Work out the finished part from the listing and answer in its coordinate system (mm). Face numbers are marked on the shaded views. A direction names the side the tool comes from. Give positions to 0.01 mm unless a question says otherwise; leave off trailing zeros. Write each loop counter-clockwise with the first axis right and the second up, starting at its lowest first coordinate (ties: lowest second). Pieces come first, ordered by that corner, then holes. Notation, with made-up numbers: (66, 41.25) -> (94, 41.25) arc R13 cw to (94, 47.25) -> close; hole circle Ø10 at (40.25, -21). An arc over 180 degrees is marked (long way). Use a Markdown table: item, result. Add a question column.
Q1. Section B-B, the plane z = 0.7 is taken. Give the vertices of the cut face in (x, y).
Q2. For the marked faces 1 and 2, determine the directions among +Z, -Z, +X, -X, +Y, -Y from which every point of the face is accessible in a straight line to the end or side of a thin tool.
Q3. Consider line 1 (Y direction, x = 13.5, z = 0.8); line 2 (Y direction, x = -13.5, z = 2.1); line 3 (Z direction, x = 1, y = -7.25). Determine where each line is inside the solid, lowest interval first.
Q4. Section D-D, the plane z = 2.5 is taken. Give the vertices of the cut face in (x, y).
Q5. Section C-C, the plane y = -1 is taken. Give the vertices of the cut face in (x, z), plus the area to 3 significant figures.
Q6. Section A-A, the plane x = -13.5 is taken. Give the vertices of the cut face in (y, z), plus the area to 3 significant figures.
Q7. This flat-tipped pin is pushed along its axis until it touches: pin 1 Ø3 at (x, y) = (-13.5, 0) entering from -Z. Where does it stop, or does it pass through?
from build123d import *

# Parameters (mm, degrees)
F0_W     = 43
F0_H     = 16
F1_DEPTH = 2
F2_R     = 3.9
F3_DEPTH = 3
F5_D     = 3.1
F6_R     = 7.5


with BuildPart() as f1:
    # F0 (on Top) → F1 (new body)
    with BuildSketch(Plane.XY):
        Rectangle(F0_W, F0_H)
    extrude(amount=F1_DEPTH)

    # F2 (on Top) → F3 (join)
    with BuildSketch(Plane.XY):
        with Locations((-13.5, 0)):
            Circle(F2_R)
        with Locations((13.5, 0)):
            Circle(F2_R)
    extrude(amount=F3_DEPTH)

    # F5 (through all)
    with Locations(Plane.XY.offset(3)):
        with Locations((-13.5, 0), (13.5, 0)):
            Hole(F5_D / 2)

    # F6
    f6_edges = [f1.edges().sort_by_distance(p)[0] for p in [
        (-21.5, -8, 1),
        (21.5, -8, 1),
        (21.5, 8, 1),
        (-21.5, 8, 1),
    ]]
    fillet(f6_edges, radius=F6_R)


solid = f1.part
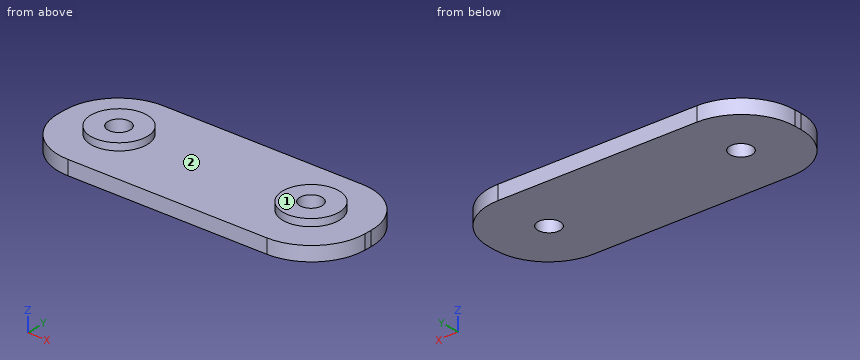
Result set:
| question | item | result |
|---|---|---|
| 1 | outline | (-21.5, -0.5) arc R7.5 ccw to (-14, -8) -> (14, -8) arc R7.5 ccw to (21.5, -0.5) -> (21.5, 0.5) arc R7.5 ccw to (14, 8) -> (-14, 8) arc R7.5 ccw to (-21.5, 0.5) -> close; hole circle Ø3.1 at (-13.5, 0); hole circle Ø3.1 at (13.5, 0) |
| 2 | face 1 | +Z, +X, -X, +Y, -Y |
| 2 | face 2 | +Z |
| 3 | line 1 | y = -8 to -1.55, 1.55 to 8 |
| 3 | line 2 | y = -3.9 to -1.55, 1.55 to 3.9 |
| 3 | line 3 | z = 0 to 2 |
| 4 | outline | circle Ø7.8 at (-13.5, 0); circle Ø7.8 at (13.5, 0); hole circle Ø3.1 at (-13.5, 0); hole circle Ø3.1 at (13.5, 0) |
| 5 | outline | (-21.48, 0) -> (-14.68, 0) -> (-14.68, 3) -> (-17.27, 3) -> (-17.27, 2) -> (-21.48, 2) -> close; (-12.32, 0) -> (12.32, 0) -> (12.32, 3) -> (9.73, 3) -> (9.73, 2) -> (-9.73, 2) -> (-9.73, 3) -> (-12.32, 3) -> close; (14.68, 0) -> (21.48, 0) -> (21.48, 2) -> (17.27, 2) -> (17.27, 3) -> (14.68, 3) -> close |
| 5 | area | 86.8 mm2 |
| 6 | outline | (-8, 0) -> (-1.55, 0) -> (-1.55, 3) -> (-3.9, 3) -> (-3.9, 2) -> (-8, 2) -> close; (1.55, 0) -> (8, 0) -> (8, 2) -> (3.9, 2) -> (3.9, 3) -> (1.55, 3) -> close |
| 6 | area | 30.5 mm2 |
| 7 | pin 1 | passes through |
